```python
from build123d import *

# Parameters (mm, degrees)
SKETCH1_R           = 46.334426
BOSS_EXTRUDE1_DEPTH = 28.68422
BOSS_EXTRUDE2_DEPTH = 23.18258
SKETCH3_R           = 16.460544738
BOSS_EXTRUDE3_DEPTH = 76.2


with BuildPart() as part:
    # Sketch1 → Boss-Extrude1 (new body)
    with BuildSketch(Plane(origin=(0, 0, 0), x_dir=(0, 0, -1), z_dir=(1, 0, 0))):
        with Locations((-75.529694, 661.049224)):
            Circle(SKETCH1_R)
    extrude(amount=BOSS_EXTRUDE1_DEPTH)

    # Sketch2 → Boss-Extrude2 (add)
    with BuildSketch(Plane(origin=(28.68422, 0, 0), x_dir=(0, 0, -1), z_dir=(1, 0, 0))):
        Polygon((-101.15042, 661.318972), (-88.573665621, 638.995898421), (-62.952939621, 638.726150421), (-49.908968, 660.779476), (-62.485722379, 683.102549579), (-88.106448379, 683.372297579), align=None)
    extrude(amount=BOSS_EXTRUDE2_DEPTH)

    # Sketch3 → Boss-Extrude3 (add)
    with BuildSketch(Plane.ZY):
        with Locations(Location((75.529694, 661.049224, 0), (0, 0, 180))):
            Circle(SKETCH3_R)
    extrude(amount=BOSS_EXTRUDE3_DEPTH)


solid = part.part
```
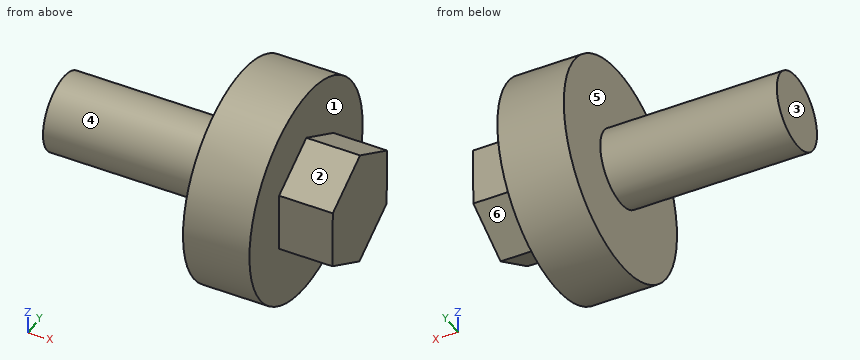
Geometry: final body of the model. Coordinates: model frame, mm. Face numbers are marked on the shaded views. A direction names the side the tool comes from. Round coordinates to 2 decimals unless told otherwise and drop trailing zeros. Loops run counter-clockwise (first coordinate to the right, second up) from the corner with the lowest first, then second, coordinate; pieces in that order, holes last.
Item 1: Reachability of the marked faces 1, 2 and 3 from +Z, -Z, +X, -X, +Y, -Y: full face, straight path, thin tool, end or side. Return the list, or none.
Checked values:
face 1: +X
face 2: +Z, +X, -Y
face 3: +Z, -Z, -X, +Y, -Y
Item 2: Section A-A, the plane x = 33. Output: boundary loops of the cut face in (y, z).
Checked values:
outline: (638.73, 62.95) - (660.78, 49.91) - (683.1, 62.49) - (683.37, 88.11) - (661.32, 101.15) - (639, 88.57) - close
Item 3: Line query: L1, parallel to X at y = 691.5, z = 83.5; L2, parallel to X at y = 650, z = 61; L3, parallel to Y at x = -7, z = 84. Output: solid intervals per line, ascending.
Checked values:
L1: x = 0 to 28.68
L2: x = 0 to 51.87
L3: y = 646.94 to 675.16
Item 4: Mould query, pull axis Y, two halves, no side actions, for the marked faces 4, 5 and 6. Classes: released by +Y, released by -Y, zero draft, split by the parting line, or undercut.
Checked values:
face 4: split by the parting line
face 5: zero draft
face 6: released by +Y
Item 5: Contact query for flat-ended pins moving along their axis: P1, Ø4, axis at y = 634.5, z = 61.5, coming from the +X side; P2, Ø12, axis at y = 644.5, z = 95, coming from the -X side; P3, Ø1.5, axis at x = 28.5, z = 97, coming from the +Y side; P4, Ø2, axis at x = 31, z = 42, coming from the +Y side. Output: stop coordinate, or through.
Checked values:
P1: stops at x = 28.68
P2: stops at x = 0
P3: stops at y = 702.49
P4: passes through
Item 6: Section C-C, the plane z = 74.5. Output: boundary loops of the cut face in (x, y).
Checked values:
outline: (-76.2, 644.62) - (0, 644.62) - (0, 614.73) - (28.68, 614.73) - (28.68, 638.85) - (51.87, 638.85) - (51.87, 683.23) - (28.68, 683.23) - (28.68, 707.37) - (0, 707.37) - (0, 677.48) - (-76.2, 677.48) - close
Item 7: Section D-D, the plane y = 631.5. Output: boundary loops of the cut face in (x, z).
Checked values:
outline: (0, 39.84) - (28.68, 39.84) - (28.68, 111.22) - (0, 111.22) - close
Item 8: Section B-B, the plane y = 659. Output: boundary loops of the cut face in (x, z).
Checked values:
outline: (-76.2, 59.2) - (0, 59.2) - (0, 29.24) - (28.68, 29.24) - (28.68, 50.96) - (51.87, 50.96) - (51.87, 99.84) - (28.68, 99.84) - (28.68, 121.82) - (0, 121.82) - (0, 91.86) - (-76.2, 91.86) - close
